Design review of the part built by this model. Coordinates are the model's own, in mm. A direction names the side the tool comes from. Round coordinates to 2 decimals unless told otherwise and drop trailing zeros. Loops run counter-clockwise (first coordinate to the right, second up) from the corner with the lowest first, then second, coordinate; pieces in that order, holes last. Notation, with made-up numbers: M 56.25,76 L 91.25,76 A15 cw 91.25,93 Z; hole C 64.5,30.25 d7. An arc over 180 degrees is marked long. One line per item, written item: value. Start each with the question number.
Item 1: We need section A-A (z = 7.5). Write out the cut boundary in (x, y).
Item 2: For line 1 along X through (y, z) = (51, 24); line 2 along X through (y, z) = (52.15, 35.5); line 3 along Y through (x, z) = (5.25, 52), list the stretches that pass through material, from the lowest coordinate up.
Item 3: Clearance check with flat-ended pins moving along their axes: pin 1 (14 mm diameter, centred on y = -11.25, z = 52, fed in from +X); pin 2 (3.5 mm diameter, centred on x = -118.5, z = 17.5, fed in from -Y); pin 3 (3.5 mm diameter, centred on y = 0, z = 52, fed in from -X). State where each tip first meets the part, or that it passes through.
Item 4: We need section C-C (y = -11.25). Write out the cut boundary in (x, z), then the cut area to 3 significant figures.
Item 5: Mouldability with a two-part tool opening along X and no side actions: class faces 3 (the flat face through (-122.5, 51, -1)), 4 (the flat face through (7.5, 9, 1)), 5 (the flat face through (-28, 52, 72)), 6 (the cylindrical face through (-117.48, 51.28, -63.67)) as released by +X, released by -X, zero draft, split by the parting line, or undercut.
Item 6: For faces 1 (the cylindrical face through (4.96, -7.19, 47.58)), 2 (the flat face through (-107.5, 51, 0)), list the 3-axis set-ups (+Z, -Z, +X, -X, +Y, -Y) from which the entire face can be reached by the end or side of a thin tool; tool diameter is ignored.
Item 7: We need section D-D (z = 64). Write out the cut boundary in (x, y), then the cut area to 4 significant figures.
Item 8: We need section B-B (x = -115). Write out the cut boundary in (y, z).
from build123d import *

# Parameters (mm, degrees)
CROQUIS1_W              = 15
CROQUIS1_H              = 144
SALIENTE_EXTRUIR1_DEPTH = 46.25
SALIENTE_EXTRUIR2_DEPTH = 7.5
CROQUIS4_W              = 77.5
CROQUIS4_H              = 22
CORTAR_EXTRUIR2_DEPTH   = 30
CROQUIS3_R              = 6
CORTAR_EXTRUIR1_DEPTH   = 15
CROQUIS5_R              = 2.5
CORTAR_EXTRUIR4_DEPTH   = 35
CROQUIS7_R              = 1.1
CORTAR_EXTRUIR6_DEPTH   = 25
CROQUIS8_W              = 144
CROQUIS8_H              = 12
CORTAR_EXTRUIR7_DEPTH   = 50
CORTAR_EXTRUIR8_DEPTH   = 190
CROQUIS10_R             = 2
CORTAR_EXTRUIR9_DEPTH   = 10
CROQUIS12_R             = 1.5
CORTAR_EXTRUIR11_DEPTH  = 10
CROQUIS13_R             = 1.5
CORTAR_EXTRUIR12_DEPTH  = 10
CORTAR_EXTRUIR13_DEPTH  = 190
CROQUIS15_R             = 1.5
CORTAR_EXTRUIR14_DEPTH  = 10
CROQUIS16_R             = 1
CORTAR_EXTRUIR15_DEPTH  = 10


with BuildPart() as part:
    # Croquis1 → Saliente-Extruir1 (new, symmetric)
    with BuildSketch(Plane(origin=(0, 0, 0), x_dir=(1, 0, 0), z_dir=(0, 1, 0))):
        Rectangle(CROQUIS1_W, CROQUIS1_H)
    extrude(amount=SALIENTE_EXTRUIR1_DEPTH, both=True)

    # Croquis2 → Saliente-Extruir2 (add, symmetric)
    with BuildSketch(Plane.XZ.offset(-46.25)):
        Polygon((-122.5, 72), (-22.5, 72), (7.5, 72), (7.5, -72), (-22.5, -72), (-122.5, -72), align=None)
    extrude(amount=SALIENTE_EXTRUIR2_DEPTH, both=True)

    # Croquis4 → Cortar-Extruir2 (cut)
    with BuildSketch(Plane(origin=(0, 53.75, 0), x_dir=(1, 0, 0), z_dir=(0, 1, 0))):
        with Locations((-68.75, 0)):
            Rectangle(CROQUIS4_W, CROQUIS4_H)
    extrude(amount=-CORTAR_EXTRUIR2_DEPTH, mode=Mode.SUBTRACT)

    # Croquis3 → Cortar-Extruir1 (cut)
    with BuildSketch(Plane.ZY.offset(7.5)):
        with Locations((52, -11.25)):
            Circle(CROQUIS3_R)
    extrude(amount=-CORTAR_EXTRUIR1_DEPTH, mode=Mode.SUBTRACT)

    # Croquis5 → Cortar-Extruir4 (cut)
    with BuildSketch(Plane(origin=(0, 53.75, 0), x_dir=(1, 0, 0), z_dir=(0, 1, 0))):
        with Locations(Location((-115, -64, 0), (0, 0, 270))):
            Circle(CROQUIS5_R)
        with Locations(Location((-115, -35.5, 0), (0, 0, 270))):
            Circle(CROQUIS5_R)
        with Locations(Location((-22.5, -35.5, 0), (0, 0, 90))):
            Circle(CROQUIS5_R)
        with Locations(Location((-22.5, -64, 0), (0, 0, 90))):
            Circle(CROQUIS5_R)
        with Locations(Location((-22.5, 64, 0), (0, 0, 270))):
            Circle(CROQUIS5_R)
        with Locations(Location((-22.5, 35.5, 0), (0, 0, 270))):
            Circle(CROQUIS5_R)
        with Locations(Location((-115, 35.5, 0), (0, 0, 90))):
            Circle(CROQUIS5_R)
        with Locations(Location((-115, 64, 0), (0, 0, 90))):
            Circle(CROQUIS5_R)
    extrude(amount=-CORTAR_EXTRUIR4_DEPTH, mode=Mode.SUBTRACT)

    # Croquis7 → Cortar-Extruir6 (cut)
    with BuildSketch(Plane(origin=(0, 53.75, 0), x_dir=(1, 0, 0), z_dir=(0, 1, 0))):
        with Locations(Location((-19, 7.9, 0), (0, 0, 270))):
            Circle(CROQUIS7_R)
        with Locations(Location((-19, -1.48, 0), (0, 0, 270))):
            Circle(CROQUIS7_R)
    extrude(amount=-CORTAR_EXTRUIR6_DEPTH, mode=Mode.SUBTRACT)

    # Croquis8 → Cortar-Extruir7 (cut)
    with BuildSketch(Plane.ZY.offset(7.5)):
        with Locations((0, -40.25)):
            Rectangle(CROQUIS8_W, CROQUIS8_H)
    extrude(amount=-CORTAR_EXTRUIR7_DEPTH, mode=Mode.SUBTRACT)

    # Croquis9 → Cortar-Extruir8 (cut)
    with BuildSketch(Plane.XY.offset(72)):
        Polygon((-7.5, -34.25), (-7.5, 38.75), (-122.5, 38.75), (-122.5, 43.75), (-2.5, 43.75), (-2.5, -34.25), align=None)
    extrude(amount=-CORTAR_EXTRUIR8_DEPTH, mode=Mode.SUBTRACT)

    # Croquis10 → Cortar-Extruir9 (cut)
    with BuildSketch(Plane.ZY.offset(2.5)):
        with Locations(Location((-20.575, -20.575, 0), (0, 0, 270))):
            Circle(CROQUIS10_R)
        with Locations(Location((-20.575, 20.575, 0), (0, 0, 270))):
            Circle(CROQUIS10_R)
        with Locations(Location((20.575, 20.575, 0), (0, 0, 270))):
            Circle(CROQUIS10_R)
        with Locations(Location((20.575, -20.575, 0), (0, 0, 270))):
            Circle(CROQUIS10_R)
    extrude(amount=-CORTAR_EXTRUIR9_DEPTH, mode=Mode.SUBTRACT)

    # Croquis12 → Cortar-Extruir11 (cut)
    with BuildSketch(Plane.XZ.offset(-43.75)):
        with Locations(Location((-12.5, 48.5, 0), (0, 0, 270))):
            Circle(CROQUIS12_R)
        with Locations(Location((-12.5, 24, 0), (0, 0, 270))):
            Circle(CROQUIS12_R)
        with Locations(Location((-27.5, 24, 0), (0, 0, 270))):
            Circle(CROQUIS12_R)
    extrude(amount=-CORTAR_EXTRUIR11_DEPTH, mode=Mode.SUBTRACT)

    # Croquis13 → Cortar-Extruir12 (cut)
    with BuildSketch(Plane(origin=(0, 53.75, 0), x_dir=(1, 0, 0), z_dir=(0, 1, 0))):
        with Locations(Location((-111, -17.5, 0), (0, 0, 270))):
            Circle(CROQUIS13_R)
        with Locations(Location((-118.5, -17.5, 0), (0, 0, 270))):
            Circle(CROQUIS13_R)
    extrude(amount=-CORTAR_EXTRUIR12_DEPTH, mode=Mode.SUBTRACT)

    # Croquis14 → Cortar-Extruir13 (cut)
    with BuildSketch(Plane.XY.offset(72)):
        Polygon((2.5, -34.25), (2.5, 48.75), (-126.1911863, 48.75), (-126.1911863, 43.75), (-2.5, 43.75), (-2.5, -34.25), align=None)
    extrude(amount=-CORTAR_EXTRUIR13_DEPTH, mode=Mode.SUBTRACT)

    # Croquis15 → Cortar-Extruir14 (cut)
    with BuildSketch(Plane(origin=(7.5, 0, 0), x_dir=(0, 0, -1), z_dir=(1, 0, 0))):
        with Locations((-52, 0)):
            Circle(CROQUIS15_R)
        with Locations((-52, 10)):
            Circle(CROQUIS15_R)
    extrude(amount=-CORTAR_EXTRUIR14_DEPTH, mode=Mode.SUBTRACT)

    # Croquis16 → Cortar-Extruir15 (cut)
    with BuildSketch(Plane(origin=(7.5, 0, 0), x_dir=(0, 0, -1), z_dir=(1, 0, 0))):
        with Locations((59, 13.75)):
            Circle(CROQUIS16_R)
        with Locations((66, 13.75)):
            Circle(CROQUIS16_R)
    extrude(amount=-CORTAR_EXTRUIR15_DEPTH, mode=Mode.SUBTRACT)


solid = part.part
A:
1. outline: M -122.5,48.75 L -107.5,48.75 L -107.5,53.75 L -122.5,53.75 Z; M -30,48.75 L 2.5,48.75 L 2.5,-34.25 L 7.5,-34.25 L 7.5,53.75 L -30,53.75 Z
2. line 1: -122.5 to -29, -26 to -14, -11 to 7.5
2. line 2: -122.5 to -117.5, -112.5 to -25, -20 to 7.5
2. line 3: -34.25 to -17.25, -5.25 to -1.5, 1.5 to 8.5, 11.5 to 53.75
3. pin 1: x = 7.5
3. pin 2: y = 48.75
3. pin 3: x = 2.5
4. outline: M 2.5,-72 L 7.5,-72 L 7.5,46 L 2.5,46 Z; M 2.5,58 L 7.5,58 L 7.5,72 L 2.5,72 Z
4. area: 660 mm2
5. face 3: released by -X
5. face 4: released by +X
5. face 5: zero draft
5. face 6: undercut
6. face 1: +X, -X
6. face 2: +Y, -Y
7. outline: M -122.5,48.75 L -117.5,48.75 L -117.5,53.75 L -122.5,53.75 Z; M -112.5,48.75 L -25,48.75 L -25,53.75 L -112.5,53.75 Z; M -20,48.75 L 2.5,48.75 L 2.5,-34.25 L 7.5,-34.25 L 7.5,53.75 L -20,53.75 Z
7. area: 1,015 mm2
8. outline: M 48.75,-72 L 53.75,-72 L 53.75,-66.5 L 48.75,-66.5 Z; M 48.75,-61.5 L 53.75,-61.5 L 53.75,-38 L 48.75,-38 Z; M 48.75,-33 L 53.75,-33 L 53.75,33 L 48.75,33 Z; M 48.75,38 L 53.75,38 L 53.75,61.5 L 48.75,61.5 Z; M 48.75,66.5 L 53.75,66.5 L 53.75,72 L 48.75,72 Z
